Part model, mm, in its own coordinate system. Face numbers are marked on the shaded views. A direction names the side the tool comes from. Give positions to 0.01 mm unless a question says otherwise; leave off trailing zeros. Loops run counter-clockwise (first coordinate to the right, second up) from the corner with the lowest first, then second, coordinate; pieces in that order, holes last. Notation, with made-up numbers: (-21.75, -14) -> (27.25, -14) arc R26 cw to (27.25, 9) -> close; hole circle Ø1 at (15, 21.5). An arc over 180 degrees is marked (long way). Write item = value, one per line.
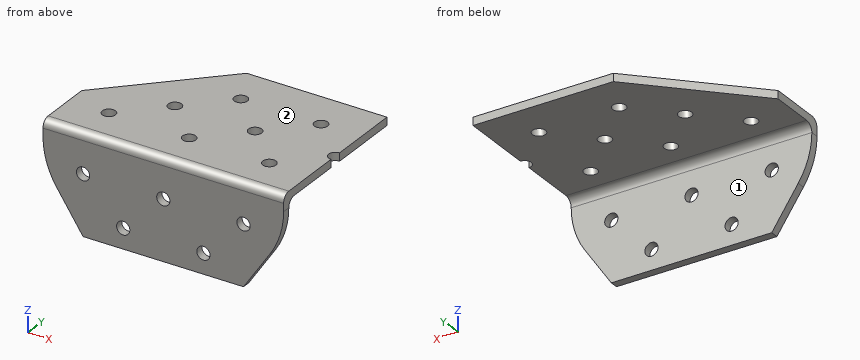
from build123d import *

# Parameters (mm, degrees)
BOSS_EXTRUDE1_DEPTH     = 76.2
SKETCH2_R               = 2.0955
CUT_EXTRUDE1_DEPTH      = 3.54
LPATTERN1_COUNT         = 3
LPATTERN1_PITCH         = 25.4
SKETCH3_R               = 2.0955
CUT_EXTRUDE2_DEPTH      = 3.54
LPATTERN2_COUNT         = 3
LPATTERN2_PITCH         = 25.4
SKETCH4_W               = 76.2
SKETCH4_H               = 19.05
CUT_EXTRUDE3_DEPTH      = 3.54
CUT_EXTRUDE5_DEPTH      = 3.54
CUT_EXTRUDE6_DEPTH      = 49.26
CUT_EXTRUDE6_DEPTH_BACK = 3.54


with BuildPart() as part:
    # Sketch1 → Boss-Extrude1 (new body)
    with BuildSketch(Plane(origin=(0, 0, 0), x_dir=(0, 0, -1), z_dir=(1, 0, 0))):
        with BuildLine():
            Line((0, 2.54), (0, 50.8))
            Line((0, 50.8), (2.54, 50.8))
            Line((2.54, 50.8), (2.54, 5.08))
            ThreePointArc((2.54, 5.08), (3.283948776, 3.283948776), (5.08, 2.54))
            Line((5.08, 2.54), (50.8, 2.54))
            Line((50.8, 2.54), (50.8, 0))
            Line((50.8, 0), (2.54, 0))
            ThreePointArc((2.54, 0), (0.743948776, 0.743948776), (0, 2.54))
        make_face()
    extrude(amount=BOSS_EXTRUDE1_DEPTH)

    # Sketch2 → Cut-Extrude1 (cut, through all)
    with BuildSketch(Plane(origin=(0, 2.54, 0), x_dir=(1, 0, 0), z_dir=(0, 1, 0))):
        with Locations((12.7, 38.0619)):
            Circle(SKETCH2_R)
        with Locations((12.7, 12.6619)):
            Circle(SKETCH2_R)
        with Locations((25.4, 25.3619)):
            Circle(SKETCH2_R)
    cut_extrude1 = extrude(amount=-CUT_EXTRUDE1_DEPTH, mode=Mode.SUBTRACT)

    # LPattern1: Cut-Extrude1 ×3
    with Locations(*[(i * LPATTERN1_PITCH, 0, 0) for i in range(1, LPATTERN1_COUNT)]):
        add(cut_extrude1, mode=Mode.SUBTRACT)

    # Sketch3 → Cut-Extrude2 (cut, through all)
    with BuildSketch(Plane(origin=(0, 0, -2.54), x_dir=(-1, 0, 0), z_dir=(0, 0, -1))):
        with Locations((-12.7, 38.1)):
            Circle(SKETCH3_R)
        with Locations((-12.7, 12.7)):
            Circle(SKETCH3_R)
        with Locations((-25.4, 25.4)):
            Circle(SKETCH3_R)
    cut_extrude2 = extrude(amount=-CUT_EXTRUDE2_DEPTH, mode=Mode.SUBTRACT)

    # LPattern2: Cut-Extrude2 ×3
    with Locations(*[(i * LPATTERN2_PITCH, 0, 0) for i in range(1, LPATTERN2_COUNT)]):
        add(cut_extrude2, mode=Mode.SUBTRACT)

    # Sketch4 → Cut-Extrude3 (cut, through all)
    with BuildSketch(Plane(origin=(0, 2.54, 0), x_dir=(1, 0, 0), z_dir=(0, 1, 0))):
        with Locations((38.1, 41.275)):
            Rectangle(SKETCH4_W, SKETCH4_H)
    extrude(amount=-CUT_EXTRUDE3_DEPTH, mode=Mode.SUBTRACT)

    # Sketch6 → Cut-Extrude5 (cut, through all)
    with BuildSketch(Plane(origin=(0, 0, -2.54), x_dir=(-1, 0, 0), z_dir=(0, 0, -1))):
        Polygon((0, 19.05), (0, 50.8), (-31.75, 50.8), align=None)
    extrude(amount=-CUT_EXTRUDE5_DEPTH, mode=Mode.SUBTRACT)

    # Sketch7 → Cut-Extrude6 (cut, two sides)
    with BuildSketch(Plane(origin=(0, 2.54, 0), x_dir=(1, 0, 0), z_dir=(0, 1, 0))) as cut_extrude6_sk:
        with BuildLine():
            Line((63.5, 31.75), (71.897549111, 19.224024233))
            ThreePointArc((71.897549111, 19.224024233), (75.100594102, 12.471963629), (76.2, 5.08))
            Line((76.2, 5.08), (76.2, 31.75))
            Line((76.2, 31.75), (63.5, 31.75))
        make_face()
        with BuildLine():
            Line((12.7, 31.75), (4.302450889, 19.224024233))
            ThreePointArc((4.302450889, 19.224024233), (1.099405898, 12.471963629), (0, 5.08))
            Line((0, 5.08), (0, 31.75))
            Line((0, 31.75), (12.7, 31.75))
        make_face()
    extrude(amount=CUT_EXTRUDE6_DEPTH, mode=Mode.SUBTRACT)
    extrude(cut_extrude6_sk.sketch, amount=-CUT_EXTRUDE6_DEPTH_BACK, mode=Mode.SUBTRACT)


solid = part.part
1) Slice it at D-D, the plane y = 25.4. List the corners of the cut face in (x, z).
Resolved:
outline = (6.35, -2.54) -> (23.3, -2.54) -> (23.3, 0) -> (6.35, 0) -> close; (27.5, -2.54) -> (48.7, -2.54) -> (48.7, 0) -> (27.5, 0) -> close; (52.9, -2.54) -> (74.1, -2.54) -> (74.1, 0) -> (52.9, 0) -> close
2) Drop flat-ended pins along their axis: P1, Ø6.5, axis at x = 12.7, z = -12.66, coming from the +Y side; P2, Ø1.5, axis at y = 7.5, z = -4, coming from the +X side; P3, Ø5, axis at x = 25.4, y = 25.4, coming from the -Z side; P4, Ø5.5, axis at x = 25.4, z = -25.36, coming from the -Y side. Give the stop position or say it passes through.
Resolved:
P1 = 2.54
P2 = through
P3 = -2.54
P4 = 0
3) Drill centre lines: line 1 along Y through (x, z) = (63.5, -1.4); line 2 along Z through (x, y) = (65, 27); line 3 along Y through (x, z) = (56.5, -25). Where is each one in solid material? Low to high. Write a range as [from, to].
Resolved:
line_1 = [0.27, 10.6], [14.8, 36], [40.2, 50.8]
line_2 = [-2.54, 0]
line_3 = [0, 2.54]
4) Slice it at A-A, the plane x = 25.4. List the corners of the cut face in (y, z), and give its area (3 significant figures).
Resolved:
outline = (0, -31.75) -> (2.54, -31.75) -> (2.54, -27.46) -> (0, -27.46) -> close; (0, -23.27) -> (2.54, -23.27) -> (2.54, -5.08) arc R2.54 cw to (5.08, -2.54) -> (23.3, -2.54) -> (23.3, 0) -> (2.54, 0) arc R2.54 ccw to (0, -2.54) -> close; (27.5, -2.54) -> (44.45, -2.54) -> (44.45, 0) -> (27.5, 0) -> close
area = 166 mm²
5) Slice it at B-B, the plane y = 12.7. List the corners of the cut face in (x, z).
Resolved:
outline = (0, -2.54) -> (10.6, -2.54) -> (10.6, 0) -> (0, 0) -> close; (14.8, -2.54) -> (36, -2.54) -> (36, 0) -> (14.8, 0) -> close; (40.2, -2.54) -> (61.4, -2.54) -> (61.4, 0) -> (40.2, 0) -> close; (65.6, -2.54) -> (76.2, -2.54) -> (76.2, 0) -> (65.6, 0) -> close
6) Slice it at C-C, the plane x = 38.1. List the corners of the cut face in (y, z), and give its area (3 significant figures).
Resolved:
outline = (0, -31.75) -> (2.54, -31.75) -> (2.54, -14.76) -> (0, -14.76) -> close; (0, -10.57) -> (2.54, -10.57) -> (2.54, -5.08) arc R2.54 cw to (5.08, -2.54) -> (10.6, -2.54) -> (10.6, 0) -> (2.54, 0) arc R2.54 ccw to (0, -2.54) -> close; (14.8, -2.54) -> (36, -2.54) -> (36, 0) -> (14.8, 0) -> close; (40.2, -2.54) -> (50.8, -2.54) -> (50.8, 0) -> (40.2, 0) -> close
area = 171 mm²
7) Which spindle directions (+Z, -Z, +X, -X, +Y, -Y) get a long thin tool onto all of the face, cutting with end or side? Do the marked faces 1 and 2. Say none if no direction does.
Resolved:
face_1 = -Z, +X, -X, +Y
face_2 = +Z, +X, -X, +Y, -Y
